from build123d import *

# Parameters (mm, degrees)
SKETCH1_R           = 1.5
BOSS_EXTRUDE1_DEPTH = 5
SKETCH2_R           = 1.5
SKETCH2_R_2         = 2.5
SKETCH2_W           = 21
SKETCH2_H           = 14
CUT_EXTRUDE1_DEPTH  = 136.576546644


with BuildPart() as part:
    # Sketch1 → Boss-Extrude1 (new body)
    with BuildSketch(Plane(origin=(0, 0, 0), x_dir=(1, 0, 0), z_dir=(0, 1, 0))):
        Polygon((64, -116), (64, -66), (70, -60), (70, -40), (65, -40), (65, -30), (70, -30), (70, 0), (-70, 0), (-70, -30), (-65, -30), (-65, -40), (-70, -40), (-70, -60), (-64, -66), (-64, -116), align=None)
        with Locations(Location((59, -5, 0), (0, 0, 270))):
            Circle(SKETCH1_R, mode=Mode.SUBTRACT)
        with Locations(Location((59, -71, 0), (0, 0, 270))):
            Circle(SKETCH1_R, mode=Mode.SUBTRACT)
        with Locations(Location((59, -111, 0), (0, 0, 270))):
            Circle(SKETCH1_R, mode=Mode.SUBTRACT)
        with Locations(Location((-59, -111, 0), (0, 0, 90))):
            Circle(SKETCH1_R, mode=Mode.SUBTRACT)
        with Locations(Location((-59, -71, 0), (0, 0, 90))):
            Circle(SKETCH1_R, mode=Mode.SUBTRACT)
        with Locations(Location((-59, -5, 0), (0, 0, 90))):
            Circle(SKETCH1_R, mode=Mode.SUBTRACT)
    extrude(amount=BOSS_EXTRUDE1_DEPTH)

    # Sketch2 → Cut-Extrude1 (cut, through all)
    with BuildSketch(Plane(origin=(0, 5, 0), x_dir=(1, 0, 0), z_dir=(0, 1, 0))):
        with Locations(Location((0, -56, 0), (0, 0, 270))):
            Circle(SKETCH2_R)
        with Locations(Location((0, -95, 0), (0, 0, 270))):
            Circle(SKETCH2_R)
        with Locations(Location((-48, -75.5, 0), (0, 0, 270))):
            Circle(SKETCH2_R_2)
        with Locations((0, -23)):
            Rectangle(SKETCH2_W, SKETCH2_H)
    extrude(amount=-CUT_EXTRUDE1_DEPTH, mode=Mode.SUBTRACT)


solid = part.part
Input: part model. Units: mm. Frame: model coordinates. A direction names the side the tool comes from. Give positions to 0.01 mm unless a question says otherwise; leave off trailing zeros. Loops run counter-clockwise (first coordinate to the right, second up) from the corner with the lowest first, then second, coordinate; pieces in that order, holes last. Notation, with made-up numbers: M 2.5,62.25 L 27.5,62.25 A26 cw 27.5,85.25 Z; hole C 77,-21 d7. An arc over 180 degrees is marked long. Use CSV: the item, a comma, the result in double quotes.
(1) Section A-A, the plane x = 59. Return loops of the section in (y, z).
Outcome:
outline,"M 0,0 L 5,0 L 5,3.5 L 0,3.5 Z; M 0,6.5 L 5,6.5 L 5,69.5 L 0,69.5 Z; M 0,72.5 L 5,72.5 L 5,109.5 L 0,109.5 Z; M 0,112.5 L 5,112.5 L 5,116 L 0,116 Z"
(2) Section B-B, the plane y = 3.2. Count the separate pieces of the cut face and the enclosed holes in it, plus the area to 3 significant figures.
Outcome:
separate pieces,"1"
enclosed holes,"10"
area,"15,100 mm²"
(3) Section C-C, the plane z = 75.5. Return loops of the section in (x, y).
Outcome:
outline,"M -64,0 L -50.5,0 L -50.5,5 L -64,5 Z; M -45.5,0 L 64,0 L 64,5 L -45.5,5 Z"
(4) Set-up query: faces 1 (the face through (-10.5, 3, 23)), 2 (the face through (-64, 2, 91)), 3 (the face through (68, 2, 40)), 4 (the face through (-65, 2, 35)). Return all of +Z, -Z, +X, -X, +Y, -Y with unobstructed straight access to the full face (end or side cutting, diameter ignored); none if empty.
Outcome:
face 1,"+Y, -Y"
face 2,"+Z, -X, +Y, -Y"
face 3,"+X, +Y, -Y"
face 4,"-X, +Y, -Y"
(5) Pin query (flat end, axial travel): P1, Ø2.5, axis at y = 3, z = 102, coming from the +X side; P2, Ø3, axis at y = 3, z = 97.5, coming from the -X side. Return the tip coordinate at first contact, or that it passes through.
Outcome:
P1,"stops at x = 64"
P2,"stops at x = -64"
(6) Material intervals for L1, parallel to Z at x = -59, y = 1.1; L2, parallel to X at y = 2.6, z = 5; L3, parallel to X at y = 2.05, z = 111, sorted ascending. Write a range as [from, to].
Outcome:
L1,"z = [0, 3.5], [6.5, 69.5], [72.5, 109.5], [112.5, 116]"
L2,"x = [-70, -60.5], [-57.5, 57.5], [60.5, 70]"
L3,"x = [-64, -60.5], [-57.5, 57.5], [60.5, 64]"
(7) Section D-D, the plane z = 5. Return loops of the section in (x, y), plus the area to 3 significant figures.
Outcome:
outline,"M -70,0 L -60.5,0 L -60.5,5 L -70,5 Z; M -57.5,0 L 57.5,0 L 57.5,5 L -57.5,5 Z; M 60.5,0 L 70,0 L 70,5 L 60.5,5 Z"
area,"670 mm²"
(8) Pull-direction query (X, two-part tool) for faces 5 (the face through (-59.07, 2.46, 112.5)), 6 (the face through (1, 2, 0)), 7 (the face through (67, 2, 63)), 8 (the face through (0, 3, 16)); classes: pulls with the +X half, pulls with the -X half, needs draft (parallel to the pull), parting line crosses it, or undercut.
Outcome:
face 5,"undercut"
face 6,"needs draft"
face 7,"pulls with the +X half"
face 8,"undercut"
